Check sheet for the modelled part. Datum: model origin and axes. Units: mm. Face numbers are marked on the shaded views. A direction names the side the tool comes from. Give positions to 0.01 mm unless a question says otherwise; leave off trailing zeros. Loops run counter-clockwise (first coordinate to the right, second up) from the corner with the lowest first, then second, coordinate; pieces in that order, holes last. Notation, with made-up numbers: M -5.5,-20 L 30.5,-20 A17 cw 30.5,0 Z; hole C 21,69 d3. An arc over 180 degrees is marked long. Use one line per item in the form item = value.
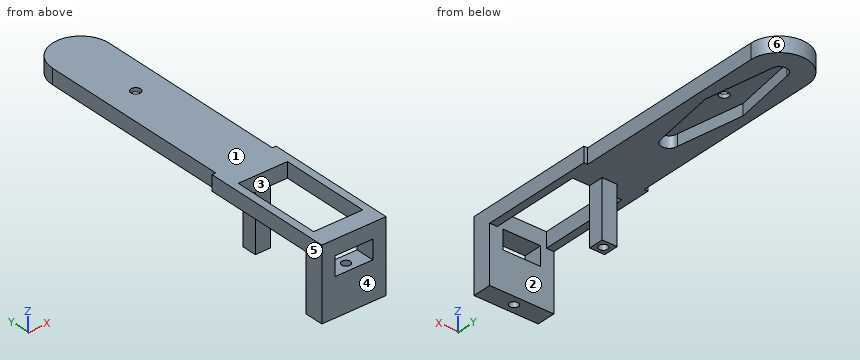
from build123d import *

# Parameters (mm, degrees)
EXTRUDE_1_DEPTH     = 4
CUT_EXTRUDE_1_DEPTH = 3
SKETCH_5_R          = 1.25
CUT_EXTRUDE_2_DEPTH = 12.4
SKETCH_6_W          = 17
SKETCH_6_H          = 35
EXTRUDE_2_DEPTH     = 4
SKETCH_7_W          = 13
SKETCH_7_H          = 24
CUT_EXTRUDE_3_DEPTH = 12.1
SKETCH_8_W          = 4
SKETCH_8_H          = 4
SKETCH_8_R          = 1.15
EXTRUDE_3_DEPTH     = 15
EXTRUDE_4_DEPTH     = 5
SKETCH_10_R         = 1.15
CUT_EXTRUDE_4_DEPTH = 12.7


with BuildPart() as part:
    # 草圖1 → 填料-伸長1 (new body)
    with BuildSketch(Plane.XY):
        with BuildLine():
            Line((7.5, 0), (7.5, 52))
            ThreePointArc((7.5, 52), (0, 59.5), (-7.5, 52))
            Line((-7.5, 52), (-7.5, 0))
            Line((-7.5, 0), (7.5, 0))
        make_face()
    extrude(amount=EXTRUDE_1_DEPTH)

    # 草圖3 → 除料-伸長1 (cut)
    with BuildSketch(Plane.XY):
        with BuildLine():
            ThreePointArc((-2.132795501, 52), (0, 54.132795501), (2.132795501, 52))
            Line((2.132795501, 52), (5, 34.5))
            Line((5, 34.5), (2.114741289, 16.658021353))
            ThreePointArc((2.114741289, 16.658021353), (-0.171540182, 14.864665347), (-2.142213835, 17))
            Line((-2.142213835, 17), (-5, 34.5))
            Line((-5, 34.5), (-2.132795501, 52))
        make_face()
    extrude(amount=CUT_EXTRUDE_1_DEPTH, mode=Mode.SUBTRACT)

    # 草圖5 → 除料-伸長2 (cut)
    with BuildSketch(Plane.XY):
        with Locations((0, 34.5)):
            Circle(SKETCH_5_R)
    extrude(amount=CUT_EXTRUDE_2_DEPTH, mode=Mode.SUBTRACT)

    # 草圖6 → 填料-伸長2 (add)
    with BuildSketch(Plane.XY):
        with Locations((0, -17.5)):
            Rectangle(SKETCH_6_W, SKETCH_6_H)
    extrude(amount=EXTRUDE_2_DEPTH)

    # 草圖7 → 除料-伸長3 (cut)
    with BuildSketch(Plane.XY):
        with Locations((0, -18)):
            Rectangle(SKETCH_7_W, SKETCH_7_H)
    extrude(amount=CUT_EXTRUDE_3_DEPTH, mode=Mode.SUBTRACT)

    # 草圖8 → 填料-伸長3 (add)
    with BuildSketch(Plane.XY):
        with Locations((0, -4)):
            Rectangle(SKETCH_8_W, SKETCH_8_H)
        with Locations((0, -4)):
            Circle(SKETCH_8_R, mode=Mode.SUBTRACT)
    extrude(amount=-EXTRUDE_3_DEPTH)

    # 草圖9 → 填料-伸長4 (add)
    with BuildSketch(Plane(origin=(0, -35, 0), x_dir=(1, 0, 0), z_dir=(0, 1, 0))):
        Polygon((-8.5, 0), (-5, 0), (-5, 5), (5, 5), (5, 0), (8.5, 0), (8.5, 15), (-8.5, 15), align=None)
    extrude(amount=EXTRUDE_4_DEPTH)

    # 草圖10 → 除料-伸長4 (cut)
    with BuildSketch(Plane(origin=(0, 0, -15), x_dir=(-1, 0, 0), z_dir=(0, 0, -1))):
        with Locations((0, -32.5)):
            Circle(SKETCH_10_R)
    extrude(amount=-CUT_EXTRUDE_4_DEPTH, mode=Mode.SUBTRACT)


solid = part.part
1) Section check B-B (y = -13.5). Record the cut outline in (x, z), then the cut area to 3 significant figures.
Evaluation:
outline = M -8.5,0 L -6.5,0 L -6.5,4 L -8.5,4 Z; M 6.5,0 L 8.5,0 L 8.5,4 L 6.5,4 Z
area = 16.0 mm^2
2) Section check C-C (x = 0.25). State how many separate pieces and enclosed holes the cut face has, then the cut area to 3 significant figures.
Evaluation:
separate_pieces = 5
enclosed_holes = 0
area = 216 mm^2
3) Set-up check for the marked faces 1 and 2: record each of +Z, -Z, +X, -X, +Y, -Y from which the full face is reachable in a straight line by a thin tool's end or side.
Evaluation:
face_1 = +Z, +X, -X, +Y, -Y
face_2 = -Z
4) Depth check by flat-ended pin: pin 1 Ø8 at (x, y) = (1.5, 29.5) entering from -Z; pin 2 Ø3 at (y, z) = (-6.5, -4) entering from +X; pin 3 Ø3 at (x, z) = (-0.5, -7) entering from +Y. Enter the tip coordinate at first touch or a pass-through.
Evaluation:
pin_1 = 0
pin_2 = 2
pin_3 = -2
5) Release check for a two-part mould opening along Y. For the marked faces 3, 4, 5 and 6 record: pulls with the +Y half, pulls with the -Y half, needs draft (parallel to the pull), parting line crosses it, or undercut.
Evaluation:
face_3 = undercut
face_4 = pulls with the -Y half
face_5 = needs draft
face_6 = pulls with the +Y half
6) Scan lines: line 1 (Y direction, x = 0, z = -8); line 2 (Y direction, x = 0, z = 3.65); line 3 (Y direction, x = 0, z = 1.75). Record each from-to range of solid material in increasing order.
Evaluation:
line_1 = -35 to -33.65, -31.35 to -30, -6 to -5.15, -2.85 to -2
line_2 = -35 to -30, -6 to 33.25, 35.75 to 59.5
line_3 = -35 to -30, -6 to 14.86, 54.13 to 59.5
7) Section check A-A (z = -3). Record the cut outline in (x, y).
Evaluation:
outline = M -8.5,-35 L -5,-35 L -5,-30 L -8.5,-30 Z; M -2,-6 L 2,-6 L 2,-2 L -2,-2 Z; M 5,-35 L 8.5,-35 L 8.5,-30 L 5,-30 Z; hole C 0,-4 d2.3
8) Section check D-D (z = 1). Record the cut outline in (x, y).
Evaluation:
outline = M -8.5,-35 L 8.5,-35 L 8.5,0 L 7.5,0 L 7.5,52 A7.5 ccw -7.5,52 L -7.5,0 L -8.5,0 Z; hole M -6.5,-30 L 6.5,-30 L 6.5,-6 L -6.5,-6 Z; hole M -5,34.5 L -2.14,17 A2.14 ccw 2.11,16.66 L 5,34.5 L 2.13,52 A2.13 ccw -2.13,52 Z
